Can you work these out from the model? Positions are in its coordinate system, mm. A direction names the side the tool comes from. Give positions to 0.01 mm unless a question says otherwise; leave off trailing zeros. Loops run counter-clockwise (first coordinate to the right, second up) from the corner with the lowest first, then second, coordinate; pieces in that order, holes last. Notation, with made-up numbers: M 62,21 L 70,21 A37 ccw 70,60 Z; hole C 39,27 d9. An arc over 180 degrees is marked long. Use CSV: the item, a comma, the result in double quotes.
from build123d import *

# Parameters (mm, degrees)
SKETCH_1_R          = 6
EXTRUDE_1_DEPTH     = 7.5
CUT_EXTRUDE_1_DEPTH = 26.75
SKETCH_4_W          = 4.5
SKETCH_4_H          = 2
CUT_EXTRUDE_2_DEPTH = 7


with BuildPart() as part:
    # 草图1 → 凸台-拉伸1 (new, symmetric)
    with BuildSketch(Plane.XY):
        with BuildLine():
            Line((-42.5, 16), (42.5, 16))
            ThreePointArc((42.5, 16), (49.571067812, 13.071067812), (52.5, 6))
            Line((52.5, 6), (52.5, -6))
            ThreePointArc((52.5, -6), (49.571067812, -13.071067812), (42.5, -16))
            Line((42.5, -16), (-42.5, -16))
            ThreePointArc((-42.5, -16), (-49.571067812, -13.071067812), (-52.5, -6))
            Line((-52.5, -6), (-52.5, 6))
            ThreePointArc((-52.5, 6), (-49.571067812, 13.071067812), (-42.5, 16))
        make_face()
        with Locations((-37.5, 0)):
            Circle(SKETCH_1_R, mode=Mode.SUBTRACT)
        with Locations((37.5, 0)):
            Circle(SKETCH_1_R, mode=Mode.SUBTRACT)
    extrude(amount=EXTRUDE_1_DEPTH, both=True)

    # 草图2 → 切除-拉伸1 (cut)
    with BuildSketch(Plane(origin=(0, 16, 0), x_dir=(1, 0, 0), z_dir=(0, 1, 0))):
        Polygon((13.15, 7.5), (11.35, 7.5), (11.35, 6.52), (9.29, 6.52), (9.29, 3.47), (11.35, 3.47), (11.35, 1.52), (9.29, 1.52), (9.29, -1.53), (11.35, -1.53), (11.35, -3.48), (9.29, -3.48), (9.29, -6.53), (11.35, -6.53), (11.35, -7.5), (13.15, -7.5), align=None)
    extrude(amount=-CUT_EXTRUDE_1_DEPTH, mode=Mode.SUBTRACT)

    # 草图4 → 切除-拉伸2 (cut)
    with BuildSketch(Plane(origin=(0, 16, 0), x_dir=(1, 0, 0), z_dir=(0, 1, 0))):
        with Locations((4.04, 4)):
            Rectangle(SKETCH_4_W, SKETCH_4_H)
        with Locations((4.04, 0)):
            Rectangle(SKETCH_4_W, SKETCH_4_H)
        with Locations((4.04, -4)):
            Rectangle(SKETCH_4_W, SKETCH_4_H)
        with Locations((18.4, 4)):
            Rectangle(SKETCH_4_W, SKETCH_4_H)
        with Locations((18.4, 0)):
            Rectangle(SKETCH_4_W, SKETCH_4_H)
        with Locations((18.4, -4)):
            Rectangle(SKETCH_4_W, SKETCH_4_H)
    extrude(amount=-CUT_EXTRUDE_2_DEPTH, mode=Mode.SUBTRACT)


solid = part.part
Q1. I want a section at B-B, the plane x = -37.5. Please give me the cut outline in (y, z).
Model answer:
outline,"M -16,-7.5 L -6,-7.5 L -6,7.5 L -16,7.5 Z; M 6,-7.5 L 16,-7.5 L 16,7.5 L 6,7.5 Z"
Q2. If we mould it in two halves opening along Z, with no side actions, what happens to faces 1 (the cylindrical face through (-49.65, 12.99, 0.11)), 2 (the flat face through (4, 9, -4)), 3 (the flat face through (10, 3, 1.53))? For each: released by +Z, released by -Z, zero draft, split by the parting line, or undercut.
Model answer:
face 1,"zero draft"
face 2,"undercut"
face 3,"undercut"
Q3. I want a section at A-A, the plane y = 0. Please give me the cut outline in (x, z).
Model answer:
outline,"M -52.5,-7.5 L -43.5,-7.5 L -43.5,7.5 L -52.5,7.5 Z; M -31.5,-7.5 L 11.35,-7.5 L 11.35,-6.52 L 9.29,-6.52 L 9.29,-3.47 L 11.35,-3.47 L 11.35,-1.52 L 9.29,-1.52 L 9.29,1.53 L 11.35,1.53 L 11.35,3.48 L 9.29,3.48 L 9.29,6.53 L 11.35,6.53 L 11.35,7.5 L -31.5,7.5 Z; M 13.15,-7.5 L 31.5,-7.5 L 31.5,7.5 L 13.15,7.5 Z; M 43.5,-7.5 L 52.5,-7.5 L 52.5,7.5 L 43.5,7.5 Z"
Q4. I want a section at C-C, the plane x = 19. Please give me the cut outline in (y, z).
Model answer:
outline,"M -16,-7.5 L 16,-7.5 L 16,-5 L 9,-5 L 9,-3 L 16,-3 L 16,-1 L 9,-1 L 9,1 L 16,1 L 16,3 L 9,3 L 9,5 L 16,5 L 16,7.5 L -16,7.5 Z"
Q5. Please list where these lines run through material, in increasing order: L1, parallel to Z at x = 10, y = 3.5; L2, parallel to Y at x = -37.5, z = 4.25; L3, parallel to X at y = 14, z = 4. Write a range as from..to.
Model answer:
L1,"-7.5..-6.52, -3.47..-1.52, 1.53..3.48, 6.53..7.5"
L2,"-16..-6, 6..16"
L3,"-48.5..1.79, 6.29..9.29, 13.15..16.15, 20.65..48.5"
Q6. I'm going to push flat-ended pins straight in: P1, Ø1, axis at y = 11.5, z = -4, coming from the -X side; P2, Ø1, axis at y = 13.5, z = 0.5, coming from the -X side; P3, Ø0.6, axis at y = 11.5, z = 0.5, coming from the -X side. Where does each tip first touch, or does it pass through?
Model answer:
P1,"x = -51.16"
P2,"x = -49.64"
P3,"x = -51.04"
Q7. For faces 4 (the flat face through (4, 13, 1)), 5 (the flat face through (11.35, 3, 2)), 6 (the cylindrical face through (-43.494, 0.264, -0.105)), which set-ups out of +Z, -Z, +X, -X, +Y, -Y let a thin tool reach every point of the face, with its end or its side?
Model answer:
face 4,"+Y"
face 5,"+Z, -Z, +Y"
face 6,"+Z, -Z"
